Check sheet for the modelled part. Datum: model origin and axes. Units: mm. A direction names the side the tool comes from. Give positions to 0.01 mm unless a question says otherwise; leave off trailing zeros. Loops run counter-clockwise (first coordinate to the right, second up) from the corner with the lowest first, then second, coordinate; pieces in that order, holes last. Notation, with made-up numbers: M 65,-1.75 L 96,-1.75 A8 cw 96,4.25 Z; hole C -30.5,-21 d7. An arc over 180 degrees is marked long. One line per question, with ' | ' between items. Start each with the question number.
from build123d import *

# Parameters (mm, degrees)
EXTRUDE_1_DEPTH = 22.5
SKETCH_2_R      = 18
EXTRUDE_2_DEPTH = 220


with BuildPart() as part:
    # Sketch 1 → Extrude 1 (new body)
    with BuildSketch(Plane.XY):
        Polygon((31.754264805, 0), (15.877132403, 27.5), (-15.877132403, 27.5), (-31.754264805, 0), (-15.877132403, -27.5), (15.877132403, -27.5), align=None)
    extrude(amount=EXTRUDE_1_DEPTH)

    # Sketch 2 → Extrude 2 (add)
    with BuildSketch(Plane.XY.offset(22.5)):
        with Locations(Location((0, 0, 0), (0, 0, 180))):
            Circle(SKETCH_2_R)
    extrude(amount=EXTRUDE_2_DEPTH)

    # Sketch 3 → Cut-Revolve 1 (revolve, cut)
    with BuildSketch(Plane(origin=(0, 0, 0), x_dir=(1, 0, 0), z_dir=(0, 1, 0)), mode=Mode.PRIVATE) as cut_revolve_1_sk:
        Polygon((31.754264805, -4), (4.6012476, 11.676801793), (47.244906426, 19.875201242), align=None)
    revolve(cut_revolve_1_sk.sketch.rotate(Axis((0, 0, -27.609458248), (0, 0, 1)), 180), axis=Axis((0, 0, -27.609458248), (0, 0, 1)), mode=Mode.SUBTRACT)


solid = part.part
Q1. Material ranges on probe 1 along Z at (x, y) = (-17, -16); probe 2 along X at (y, z) = (-16, 76.5); probe 3 along X at (y, z) = (-1, 26), recorded low to high. Write a range as from..to.
Q2. Cross-section at A-A (x = 0). Record the cut outline in (y, z).
Q3. Depth check by flat-ended pin: P1, Ø4, axis at y = 10.5, z = 140.5, coming from the -X side; P2, Ø10, axis at y = -20, z = 65.5, coming from the -X side; P3, Ø5, axis at y = -8.5, z = 174, coming from the +X side. Enter the tip coordinate at first touch or a pass-through.
Q4. Cross-section at B-B (z = 35). Record the cut outline in (x, y).
Q5. Access from +Z, -Z, +X, -X, +Y, -Y to the whole of each face (thin tool, end or side, straight path). Record for faces 1 (the flat face through (0, -27.5, 12)), 2 (the cylindrical face through (13.267, -12.165, 130.96)).
Solved:
1) probe 1: z = 0..22.5 | probe 2: x = -8.25..8.25 | probe 3: x = -17.97..17.97
2) outline: M -27.5,1.54 L -24.83,0 L 24.83,0 L 27.5,1.54 L 27.5,22.5 L 18,22.5 L 18,242.5 L -18,242.5 L -18,22.5 L -27.5,22.5 Z
3) P1: stops at x = -15.87 | P2: stops at x = -9.95 | P3: stops at x = 16.97
4) outline: C 0,0 d36
5) face 1: +Z, -Z, +X, -X, -Y | face 2: +Z
